For this review, take the finished solid that the model builds, in its own axes (mm). Round coordinates to 2 decimals unless told otherwise and drop trailing zeros. Write each loop counter-clockwise with the first axis right and the second up, starting at its lowest first coordinate (ties: lowest second). Pieces come first, ordered by that corner, then holes. Notation, with made-up numbers: (-14.75, 45.5) -> (2.25, 45.5) arc R14 ccw to (2.25, 49.5) -> close; hole circle Ø6 at (5.25, -37.5). An arc over 180 degrees is marked (long way). Answer in a Markdown table with one row per item. Add a question column.
```python
from build123d import *

# Parameters (mm, degrees)
SKETCH1_R           = 2.25
BOSS_EXTRUDE1_DEPTH = 4


with BuildPart() as part:
    # Sketch1 → Boss-Extrude1 (new body)
    with BuildSketch(Plane(origin=(0, 0, 0), x_dir=(1, 0, 0), z_dir=(0, 1, 0))):
        Polygon((0, 4.618802154), (-4, 2.309401077), (-4, -2.309401077), (0, -4.618802154), (4, -2.309401077), (4, 2.309401077), align=None)
        with Locations(Location((0, 0, 0), (0, 0, 270))):
            Circle(SKETCH1_R, mode=Mode.SUBTRACT)
    extrude(amount=BOSS_EXTRUDE1_DEPTH)

    # Sketch2 → Cut-Revolve1 (revolve, cut)
    with BuildSketch(Plane(origin=(0, 0, 0), x_dir=(0, 0, -1), z_dir=(1, 0, 0))):
        Polygon((-5.075475812, 3.142855419), (-2.444726969, 4.683764438), (-4.731695124, 4.838553625), align=None)
        Polygon((-4.731695124, -0.838553625), (-5.075475812, 0.857144581), (-2.444726969, -0.683764438), align=None)
    revolve(axis=Axis((0, 4.212316803, 0), (0, -1, 0)), mode=Mode.SUBTRACT)


solid = part.part
```
1. We need section C-C (y = 3.55). Write out the cut boundary in (x, z), plus the area to 3 significant figures.
2. For L1, parallel to X at y = 2.8, z = 0; L2, parallel to X at y = 2.3, z = 1.5; L3, parallel to X at y = 0.4, z = -3.5, list the stretches that pass through material, from the lowest coordinate up. Write a range as [from, to].
3. Clearance check with a flat-ended pin moving along its axis: pin 1 Ø2.5 at (x, z) = (0, 0) entering from +Y. State where the tip first meets the part, or that it passes through.
4. We need section B-B (y = 2.55). Write out the cut boundary in (x, z).
5. We need section A-A (z = 0). Write out the cut boundary in (x, y), plus the area to 3 significant figures.
6. The part is to be moulded in two halves that separate along Z. For faces 1 (the flat face through (-1.97, 1.98, -3.48)), 2 (the flat face through (-4, 2, 0)), 3 (the cylindrical face through (0.676, 1.972, 2.146)), say which applies: pulls with the +Z half, pulls with the -Z half, needs draft (parallel to the pull), parting line crosses it, or undercut.
Response:
| question | item | result |
|---|---|---|
| 1 | outline | (-4, -1.79) arc R4.38 ccw to (-3.55, -2.57) -> (-0.45, -4.36) arc R4.38 ccw to (0.45, -4.36) -> (3.55, -2.57) arc R4.38 ccw to (4, -1.79) -> (4, 1.79) arc R4.38 ccw to (3.55, 2.57) -> (0.45, 4.36) arc R4.38 ccw to (-0.45, 4.36) -> (-3.55, 2.57) arc R4.38 ccw to (-4, 1.79) -> close; hole circle Ø4.5 at (0, 0) |
| 1 | area | 38.9 mm2 |
| 2 | L1 | [-4, -2.25], [2.25, 4] |
| 2 | L2 | [-4, -1.68], [1.68, 4] |
| 2 | L3 | [-1.94, 1.94] |
| 3 | pin 1 | through |
| 4 | outline | (-4, -2.31) -> (0, -4.62) -> (4, -2.31) -> (4, 2.31) -> (0, 4.62) -> (-4, 2.31) -> close; hole circle Ø4.5 at (0, 0) |
| 5 | outline | (-4, 0.23) -> (-3.61, 0) -> (-2.25, 0) -> (-2.25, 4) -> (-3.61, 4) -> (-4, 3.77) -> close; (2.25, 0) -> (3.61, 0) -> (4, 0.23) -> (4, 3.77) -> (3.61, 4) -> (2.25, 4) -> close |
| 5 | area | 13.8 mm2 |
| 6 | face 1 | pulls with the -Z half |
| 6 | face 2 | needs draft |
| 6 | face 3 | undercut |
